from build123d import *

# Parameters (mm, degrees)
SKETCH1_W           = 26.5
SKETCH1_H           = 6
BOSS_EXTRUDE1_DEPTH = 17
SKETCH2_R           = 1.5
CUT_EXTRUDE1_DEPTH  = 1
SKETCH3_R           = 1.3
CUT_EXTRUDE2_DEPTH  = 32.878676259
SKETCH4_R           = 4
CUT_EXTRUDE3_DEPTH  = 33.050741021
SKETCH5_R           = 2.5
CUT_EXTRUDE4_DEPTH  = 1.5
SKETCH6_R           = 1.5
CUT_EXTRUDE8_DEPTH  = 1
SKETCH7_R           = 1.3
CUT_EXTRUDE9_DEPTH  = 32.678068123
CUT_EXTRUDE10_START = -1
SKETCH8_R           = 2.5
CUT_EXTRUDE10_DEPTH = 1
CUT_EXTRUDE11_START = -1
SKETCH9_R           = 1.5
CUT_EXTRUDE11_DEPTH = 1
SKETCH10_R          = 5.5
SKETCH10_R_2        = 4
BOSS_EXTRUDE2_DEPTH = 3.5
SKETCH11_R          = 3
SKETCH11_R_2        = 1.3
BOSS_EXTRUDE4_DEPTH = 2
CUT_EXTRUDE12_START = -1
SKETCH12_R          = 1.5
CUT_EXTRUDE12_DEPTH = 1
SKETCH17_W          = 2
SKETCH17_H          = 6
BOSS_EXTRUDE6_DEPTH = 1.5
SKETCH18_R          = 1
CUT_EXTRUDE17_DEPTH = 33.050741021
CHAMFER2_SIZE       = 5
CHAMFER2_SIZE2      = 3.5
FILLET11_R          = 3
BOSS_EXTRUDE7_DEPTH = 2
CUT_EXTRUDE19_DEPTH = 33.050741021
FILLET13_R          = 5
FILLET14_R          = 3
FILLET15_R          = 3


with BuildPart() as part:
    # Sketch1 → Boss-Extrude1 (new body)
    with BuildSketch(Plane(origin=(0, 0, 0), x_dir=(1, 0, 0), z_dir=(0, 1, 0))):
        with Locations((13.25, 3)):
            Rectangle(SKETCH1_W, SKETCH1_H)
    extrude(amount=BOSS_EXTRUDE1_DEPTH)

    # Sketch2 → Cut-Extrude1 (cut)
    with BuildSketch(Plane.XY):
        with Locations((12.5, 5.5)):
            Circle(SKETCH2_R)
    extrude(amount=-CUT_EXTRUDE1_DEPTH, mode=Mode.SUBTRACT)

    # Sketch3 → Cut-Extrude2 (cut, through all)
    with BuildSketch(Plane.XY.offset(-1)):
        with Locations((12.5, 5.5)):
            Circle(SKETCH3_R)
    extrude(amount=-CUT_EXTRUDE2_DEPTH, mode=Mode.SUBTRACT)

    # Sketch4 → Cut-Extrude3 (cut, through all)
    with BuildSketch(Plane.XY):
        with Locations((19.208203932, 11.5)):
            Circle(SKETCH4_R)
    extrude(amount=-CUT_EXTRUDE3_DEPTH, mode=Mode.SUBTRACT)

    # Sketch5 → Cut-Extrude4 (cut)
    with BuildSketch(Plane.XY):
        with Locations((3.5, 5.5)):
            Circle(SKETCH5_R)
    extrude(amount=-CUT_EXTRUDE4_DEPTH, mode=Mode.SUBTRACT)

    # Sketch6 → Cut-Extrude8 (cut)
    with BuildSketch(Plane.XY.offset(-1.5)):
        with Locations((3.5, 5.5)):
            Circle(SKETCH6_R)
    extrude(amount=-CUT_EXTRUDE8_DEPTH, mode=Mode.SUBTRACT)

    # Sketch7 → Cut-Extrude9 (cut, through all)
    with BuildSketch(Plane.XY.offset(-2.5)):
        with Locations((3.5, 5.5)):
            Circle(SKETCH7_R)
    extrude(amount=-CUT_EXTRUDE9_DEPTH, mode=Mode.SUBTRACT)

    # Sketch8 → Cut-Extrude10 (cut)
    with BuildSketch(Plane(origin=(0, 0, -6), x_dir=(-1, 0, 0), z_dir=(0, 0, -1)).offset(CUT_EXTRUDE10_START)):
        with Locations(Location((-3.5, 5.5, 0), (0, 0, 180))):
            Circle(SKETCH8_R)
    extrude(amount=CUT_EXTRUDE10_DEPTH, mode=Mode.SUBTRACT)

    # Sketch9 → Cut-Extrude11 (cut)
    with BuildSketch(Plane(origin=(0, 0, -5), x_dir=(-1, 0, 0), z_dir=(0, 0, -1)).offset(CUT_EXTRUDE11_START)):
        with Locations(Location((-3.5, 5.5, 0), (0, 0, 180))):
            Circle(SKETCH9_R)
    extrude(amount=CUT_EXTRUDE11_DEPTH, mode=Mode.SUBTRACT)

    # Sketch10 → Boss-Extrude2 (add)
    with BuildSketch(Plane(origin=(0, 0, -6), x_dir=(-1, 0, 0), z_dir=(0, 0, -1))):
        with Locations(Location((-19.208203932, 11.5, 0), (0, 0, 90))):
            Circle(SKETCH10_R)
        with Locations(Location((-19.208203932, 11.5, 0), (0, 0, 180))):
            Circle(SKETCH10_R_2, mode=Mode.SUBTRACT)
    extrude(amount=BOSS_EXTRUDE2_DEPTH)

    # Sketch11 → Boss-Extrude4 (add)
    with BuildSketch(Plane(origin=(0, 0, -6), x_dir=(-1, 0, 0), z_dir=(0, 0, -1))):
        with Locations(Location((-12.5, 5.5, 0), (0, 0, 180))):
            Circle(SKETCH11_R)
        with Locations(Location((-12.5, 5.5, 0), (0, 0, 180))):
            Circle(SKETCH11_R_2, mode=Mode.SUBTRACT)
    extrude(amount=BOSS_EXTRUDE4_DEPTH)

    # Sketch12 → Cut-Extrude12 (cut)
    with BuildSketch(Plane(origin=(0, 0, -8), x_dir=(-1, 0, 0), z_dir=(0, 0, -1)).offset(CUT_EXTRUDE12_START)):
        with Locations(Location((-12.5, 5.5, 0), (0, 0, 180))):
            Circle(SKETCH12_R)
    extrude(amount=CUT_EXTRUDE12_DEPTH, mode=Mode.SUBTRACT)

    # Sketch17 → Boss-Extrude6 (add)
    with BuildSketch(Plane.XZ):
        with Locations((6, -3)):
            Rectangle(SKETCH17_W, SKETCH17_H)
        with Locations((20.5, -3)):
            Rectangle(SKETCH17_W, SKETCH17_H)
    extrude(amount=BOSS_EXTRUDE6_DEPTH)

    # Sketch18 → Cut-Extrude17 (cut, through all)
    with BuildSketch(Plane(origin=(0, 0, -6), x_dir=(-1, 0, 0), z_dir=(0, 0, -1))):
        with Locations((-22.5, 0)):
            Circle(SKETCH18_R)
        with Locations((-18.5, 0)):
            Circle(SKETCH18_R)
        with Locations((-8, 0)):
            Circle(SKETCH18_R)
        with Locations((-4, 0)):
            Circle(SKETCH18_R)
    extrude(amount=-CUT_EXTRUDE17_DEPTH, mode=Mode.SUBTRACT)

    # Chamfer2
    chamfer2_edges = [part.edges().sort_by_distance(p)[0] for p in [
        (26.5, 17, -3),
    ]]
    chamfer2_side = [part.faces().sort_by_distance(p)[0] for p in [
        (26.5, 8.5, -3),
    ]]
    chamfer(chamfer2_edges, length=CHAMFER2_SIZE, length2=CHAMFER2_SIZE2, reference=chamfer2_side[0])

    # Fillet11
    fillet11_edges = [part.edges().sort_by_distance(p)[0] for p in [
        (23, 17, -3),
        (26.5, 12, -3),
    ]]
    fillet(fillet11_edges, radius=FILLET11_R)

    # Sketch19 → Boss-Extrude7 (add)
    with BuildSketch(Plane(origin=(0, 0, -6), x_dir=(-1, 0, 0), z_dir=(0, 0, -1))):
        with BuildLine():
            Line((-14.547099294, 14.419606745), (-9.957579288, 7.09251277))
            ThreePointArc((-9.957579288, 7.09251277), (-14.736067977, 7.5), (-13.800160725, 2.796376119))
            Line((-13.800160725, 2.796376119), (-21.591831928, 6.543356218))
            ThreePointArc((-21.591831928, 6.543356218), (-15.108745974, 7.833333333), (-14.547099294, 14.419606745))
        make_face()
    extrude(amount=BOSS_EXTRUDE7_DEPTH)

    # Sketch20 → Cut-Extrude19 (cut, through all)
    with BuildSketch(Plane(origin=(0, 0, -6), x_dir=(-1, 0, 0), z_dir=(0, 0, -1))):
        Polygon((0, 17), (-14.011012575, 17), (-9, 9), (0, 9), align=None)
    extrude(amount=-CUT_EXTRUDE19_DEPTH, mode=Mode.SUBTRACT)

    # Fillet13
    fillet13_edges = [part.edges().sort_by_distance(p)[0] for p in [
        (14.011012575, 17, -3),
    ]]
    fillet(fillet13_edges, radius=FILLET13_R)

    # Fillet14
    fillet14_edges = [part.edges().sort_by_distance(p)[0] for p in [
        (9, 9, -3),
    ]]
    fillet(fillet14_edges, radius=FILLET14_R)

    # Fillet15
    fillet15_edges = [part.edges().sort_by_distance(p)[0] for p in [
        (0, 9, -3),
    ]]
    fillet(fillet15_edges, radius=FILLET15_R)


solid = part.part
Geometry: final body of the model. Coordinates: model frame, mm. A direction names the side the tool comes from. Round coordinates to 2 decimals unless told otherwise and drop trailing zeros. Write each loop counter-clockwise with the first axis right and the second up, starting at its lowest first coordinate (ties: lowest second). Pieces come first, ordered by that corner, then holes. Notation, with made-up numbers: M 85.25,-8 L 109.25,-8 A25 cw 109.25,8 Z; hole C -27,3.5 d10. An arc over 180 degrees is marked long. Write item = value, one per line.
Item 1: Section query C-C on x = 3.5. Return loops of the section in (y, z), then the cut area to 3 significant figures.
Findings:
outline = M 0.87,-6 L 3,-6 L 3,-5 L 4,-5 L 4,-4 L 4.2,-4 L 4.2,-2.5 L 4,-2.5 L 4,-1.5 L 3,-1.5 L 3,0 L 0.87,0 Z; M 6.8,-4 L 7,-4 L 7,-5 L 8,-5 L 8,-6 L 9,-6 L 9,0 L 8,0 L 8,-1.5 L 7,-1.5 L 7,-2.5 L 6.8,-2.5 Z
area = 26.4 mm^2
Item 2: Access query for faces 1 (the face through (13, 0, -3)), 2 (the face through (1, 0, -3)), 3 (the face through (4.886, 4.925, -1.993)). Directions: +Z, -Z, +X, -X, +Y, -Y. A direction counts if a zero-diameter tool reaches every point of the face in a straight line with its end or side. Return the directions, or none.
Findings:
face_1 = +Z, -Z, -Y
face_2 = +Z, -Z, -X, -Y
face_3 = +Z
Item 3: Pull-direction query (Y, two-part tool) for faces 4 (the face through (5, -1, -3)), 5 (the face through (17.641, 4.644, -6.986)), 6 (the face through (5, 4, -1.5)), 7 (the face through (5.885, 6.251, -0.74)); classes: pulls with the +Y half, pulls with the -Y half, needs draft (parallel to the pull), parting line crosses it, or undercut.
Findings:
face_4 = needs draft
face_5 = pulls with the -Y half
face_6 = undercut
face_7 = undercut
Item 4: Section query B-B on y = 12.25. Return loops of the section in (x, z), then the cut area to 3 significant figures.
Findings:
outline = M 11.04,-6 L 13.19,-6 L 13.19,-8 L 13.76,-8 L 13.76,-9.5 L 15.28,-9.5 L 15.28,0 L 11.04,0 Z; M 23.14,-9.5 L 24.66,-9.5 L 24.66,-6 L 26.25,-6 L 26.25,0 L 23.14,0 Z
area = 55.9 mm^2
Item 5: Material intervals for line 1 along X through (y, z) = (0.75, -0.5); line 2 along X through (y, z) = (5.75, -4.75); line 3 along Z through (x, y) = (14.25, 2.25), sorted ascending. Write a range as [from, to].
Findings:
line_1 = [0, 3.34], [4.66, 7.34], [8.66, 17.84], [19.16, 21.84], [23.16, 26.5]
line_2 = [0, 2.02], [4.98, 11.22], [13.78, 26.5]
line_3 = [-6, 0]
Item 6: Section query D-D on y = 1.75. Return loops of the section in (x, z).
Findings:
outline = M 0,-6 L 26.5,-6 L 26.5,0 L 0,0 Z
Item 7: Pin query (flat end, axial travel): P1, Ø1.8, axis at x = 3.5, y = 5.5, coming from the -Z side; P2, Ø6, axis at x = 3.5, y = 5.5, coming from the -Z side; P3, Ø3.5, axis at x = 4.5, z = -2, coming from the +Y side; P4, Ø0.9, axis at x = 24.5, z = -3, coming from the -Y side. Return the tip coordinate at first contact, or that it passes through.
Findings:
P1 = through
P2 = -6
P3 = 9
P4 = 0
Item 8: Section query A-A on x = 18.5. Return loops of the section in (y, z).
Findings:
outline = M 1,-6 L 5.06,-6 L 5.06,-8 L 6.05,-8 L 6.05,-9.5 L 7.56,-9.5 L 7.56,0 L 1,0 Z; M 15.44,-9.5 L 16.95,-9.5 L 16.95,-6 L 17,-6 L 17,0 L 15.44,0 Z
